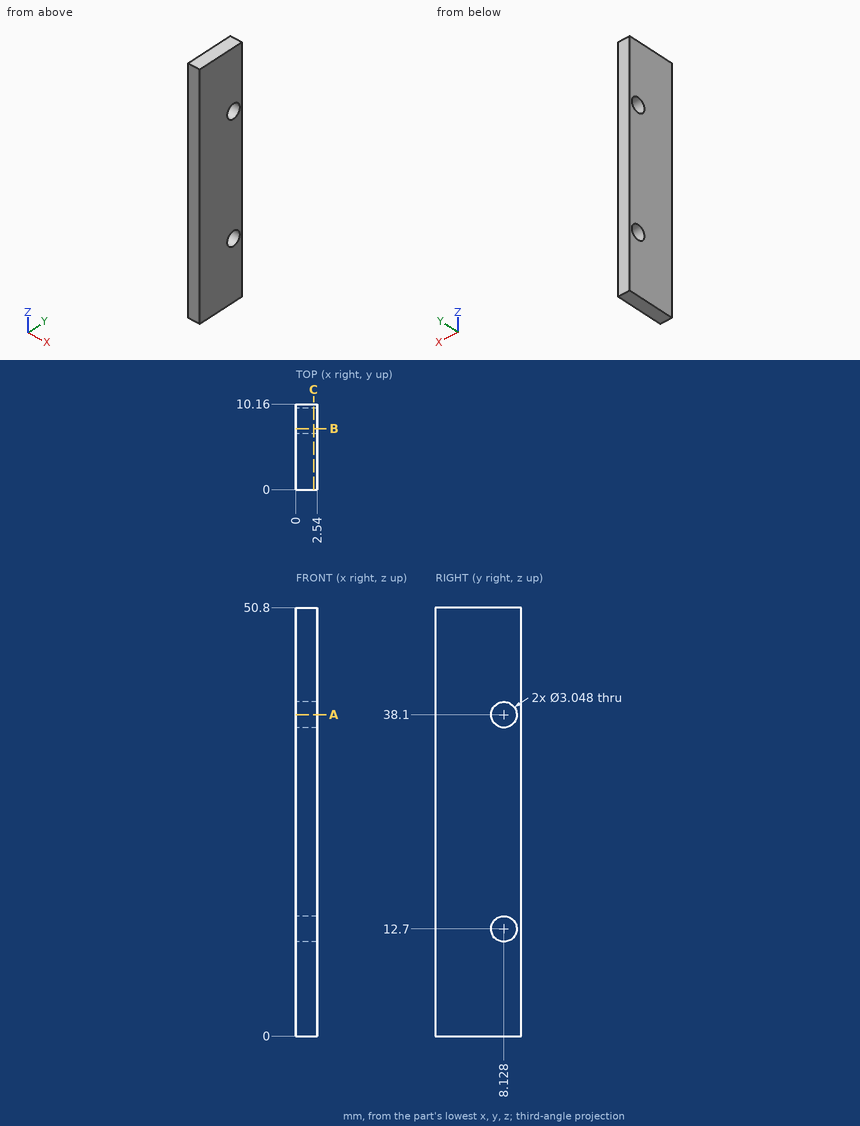
Study the drawing (mm; zero at the part's minimum x, y, z) and answer. Coordinates: 2 decimals unless noted, no trailing zeros. Write each loop counter-clockwise with the first axis right and the second up, starting at its lowest first coordinate (ties: lowest second). Pieces come first, ordered by that corner, then holes. Notation, with made-up numbers: (30, 45) - (48, 45) arc R27 cw to (48, 73) - close; hole circle Ø9 at (0, 44). An arc over 180 degrees is marked (long way). One line per item, written item: value.
1) Find section B-B (y = 7.25). Give the vertices of the cut face in (x, z).
Geometry check:
outline: (0, 0) - (2.54, 0) - (2.54, 11.45) - (0, 11.45) - close; (0, 13.95) - (2.54, 13.95) - (2.54, 36.85) - (0, 36.85) - close; (0, 39.35) - (2.54, 39.35) - (2.54, 50.8) - (0, 50.8) - close
2) Find section A-A (z = 38.1). Give the vertices of the cut face in (x, y), and give its area (3 significant figures).
Geometry check:
outline: (0, 0) - (2.54, 0) - (2.54, 6.6) - (0, 6.6) - close; (0, 9.65) - (2.54, 9.65) - (2.54, 10.16) - (0, 10.16) - close
area: 18.1 mm2
3) Find section C-C (x = 2.1). Give the vertices of the cut face in (y, z), and give its area (3 significant figures).
Geometry check:
outline: (0, 0) - (10.16, 0) - (10.16, 50.8) - (0, 50.8) - close; hole circle Ø3.05 at (8.13, 12.7); hole circle Ø3.05 at (8.13, 38.1)
area: 502 mm2
4) Consider line 1 along Y through (x, z) = (1.4, 12.7); line 2 along Z through (x, y) = (0.4, 9); line 3 along Z through (x, y) = (0.3, 9.5). Determine where each line is inside the solid, lowest interval first. Write a range as from..to.
Geometry check:
line 1: y = 0..6.6, 9.65..10.16
line 2: z = 0..11.45, 13.95..36.85, 39.35..50.8
line 3: z = 0..12.04, 13.36..37.44, 38.76..50.8
